Part model, mm, in its own coordinate system. A direction names the side the tool comes from. Coordinates: 2 decimals unless noted, no trailing zeros.
```python
from build123d import *

# Parameters (mm, degrees)
F0_W             = 12.5
F0_H             = 25
F1_DEPTH         = 100
F2_W             = 2.28
F2_H             = 3.25
F3_DEPTH         = 200
F3_COPIES_COUNT  = 2
F3_COPIES_ANGLE  = 90
F3_COPIES1_COUNT = 2
F3_COPIES1_ANGLE = 270
F5_R             = 1
F7_R             = 2.5374832391
F8_DEPTH         = 200


# Not quite as in the source:
# - a pattern or mirror of a feature is missing from the dataset's text; its kind, count and spacing are read off the source's solid


with BuildPart() as f1:
    # F0 (on Right) → F1 (new body, symmetric)
    with BuildSketch(Plane.YZ):
        with Locations((-6.25, 12.5)):
            Rectangle(F0_W, F0_H)
        Polygon((0, 0), (12.5, 0), (12.5, 9.25), (10.22, 9.25), (10.22, 5.155), (4.38, 5.155), (4.38, 9.25), (4.38, 10.995), (4.38, 14.005), (4.38, 15.75), (4.38, 19.845), (10.22, 19.845), (10.22, 15.75), (12.5, 15.75), (12.5, 25), (0, 25), align=None)
        Polygon((10.22, 5.155), (6.125, 9.25), (4.38, 9.25), (4.38, 5.155), align=None)
        Polygon((4.38, 9.25), (6.125, 9.25), (4.38, 10.995), align=None)
        Polygon((4.38, 14.005), (6.125, 15.75), (4.38, 15.75), align=None)
        Polygon((4.38, 15.75), (6.125, 15.75), (10.22, 19.845), (4.38, 19.845), align=None)
    extrude(amount=F1_DEPTH, both=True)

    # F2 (on face) → F3 (cut, through all)
    with BuildSketch(Plane(origin=(-100, 0, 0), x_dir=(0, -1, 0), z_dir=(-1, 0, 0))):
        with Locations((11.36, 10.875)):
            Rectangle(F2_W, F2_H)
        with BuildLine():
            Line((0, 15.0374832391), (0, 9.9625167609))
            ThreePointArc((0, 9.9625167609), (1.7942716055, 10.7057283945), (2.5374832391, 12.5))
            ThreePointArc((2.5374832391, 12.5), (1.7942716055, 14.2942716055), (0, 15.0374832391))
        make_face()
        with Locations((11.36, 14.125)):
            Rectangle(F2_W, F2_H)
        Polygon((10.22, 5.155), (10.22, 9.25), (6.125, 9.25), align=None)
        Polygon((6.125, 9.25), (10.22, 9.25), (10.22, 12.5), (10.22, 15.75), (6.125, 15.75), (4.38, 14.005), (4.38, 10.995), align=None)
        Polygon((6.125, 15.75), (10.22, 15.75), (10.22, 19.845), align=None)
    f3 = extrude(amount=-F3_DEPTH, mode=Mode.SUBTRACT)

    # F3_copies: F3 ×2 about axis
    f3_copies_axis = Axis((0, 0, 12.5), (1, 0, 0))
    for i in range(1, F3_COPIES_COUNT):
        add(f3.rotate(f3_copies_axis, i * F3_COPIES_ANGLE / (F3_COPIES_COUNT - 1)), mode=Mode.SUBTRACT)

    # F3_copies1: F3 ×2 about axis
    f3_copies1_axis = Axis((0, 0, 12.5), (1, 0, 0))
    for i in range(1, F3_COPIES1_COUNT):
        add(f3.rotate(f3_copies1_axis, i * F3_COPIES1_ANGLE / (F3_COPIES1_COUNT - 1)), mode=Mode.SUBTRACT)

    # F5
    f5_edges = [f1.edges().sort_by_distance(p)[0] for p in [
        (0, -4.38, 14.005),
        (0, -4.38, 10.995),
        (0, -10.22, 19.845),
        (0, -10.22, 15.75),
        (0, -12.5, 15.75),
        (0, -12.5, 9.25),
        (0, -10.22, 9.25),
        (0, -10.22, 5.155),
        (0, 12.5, 25),
        (0, -12.5, 25),
        (0, -12.5, 0),
        (0, 12.5, 0),
        (0, 10.22, 19.845),
        (0, 10.22, 15.75),
        (0, 4.38, 14.005),
        (0, 4.38, 10.995),
        (0, 10.22, 5.155),
        (0, 10.22, 9.25),
        (0, 12.5, 9.25),
        (0, 3.25, 0),
        (0, 3.25, 2.28),
        (0, 7.345, 2.28),
        (0, 1.505, 8.12),
        (0, -1.505, 8.12),
        (0, -7.345, 2.28),
        (0, -3.25, 2.28),
        (0, -3.25, 0),
        (0, -3.25, 22.72),
        (0, -3.25, 25),
        (0, -7.345, 22.72),
        (0, -1.505, 16.88),
        (0, 1.505, 16.88),
        (0, 7.345, 22.72),
        (0, 3.25, 22.72),
        (0, 3.25, 25),
        (0, 12.5, 15.75),
    ]]
    fillet(f5_edges, radius=F5_R)

    # F7 (on face) → F8 (cut, through all)
    with BuildSketch(Plane(origin=(-100, 0, 0), x_dir=(0, -1, 0), z_dir=(-1, 0, 0))):
        with BuildLine():
            ThreePointArc((0, 9.5939878347), (2.0548609083, 10.4451390917), (2.9060121653, 12.5))
            ThreePointArc((2.9060121653, 12.5), (2.0548609083, 14.5548609083), (0, 15.4060121653))
            ThreePointArc((0, 15.4060121653), (-2.0548609083, 14.5548609083), (-2.9060121653, 12.5))
            ThreePointArc((-2.9060121653, 12.5), (-2.0548609083, 10.4451390917), (0, 9.5939878347))
        make_face()
        with Locations((0, 12.5)):
            Circle(F7_R, mode=Mode.SUBTRACT)
    extrude(amount=-F8_DEPTH, mode=Mode.SUBTRACT)


solid = f1.part
```
Q1. Tool access for faces 1 (the flat face through (-1.4, -6.566, 8.809)), 2 (the flat face through (1, 8, 25)): list every direction of +Z, -Z, +X, -X, +Y, -Y with a clear straight run to the whole face (end or side of a thin tool).
Q2. Probe line 1 (Y direction, x = -34.5, z = 21) (3 decimals); line 2 (Z direction, x = 59.5, y = 5.75) (3 decimals); line 3 (Y direction, x = -13, z = 23.5). List the from-to ranges inside material, lowest first.
Q3. Drop flat-ended pins along their axis: P1, Ø1.7, axis at x = 39, z = 12.5, coming from the -Y side; P2, Ø1.1, axis at x = -32, z = 13, coming from the +Y side; P3, Ø1.1, axis at x = 0, y = 0, coming from the +Z side. Give the stop position or say it passes through.
Q4. Mould opens along Y. For faces 3 (the flat face through (1, -12.5, 5)), 4 (the flat face through (100, 3, 10)), 5 (the flat face through (-1.4, 3.691, 5.934)) say: released by +Y, released by -Y, zero draft, split by the parting line, or undercut.
Checked values:
1. face 1: +X, -X
1. face 2: +Z, +X, -X, +Y, -Y
2. line 1: y = -12.5 to -5.625, 5.625 to 12.5
2. line 2: z = 0 to 2.707, 3.853 to 9.625, 15.375 to 21.147, 22.293 to 25
2. line 3: y = -12.5 to -3.27, 3.27 to 12.5
3. P1: stops at y = -4.38
3. P2: stops at y = 4.38
3. P3: stops at z = 16.88
4. face 3: released by -Y
4. face 4: zero draft
4. face 5: undercut
